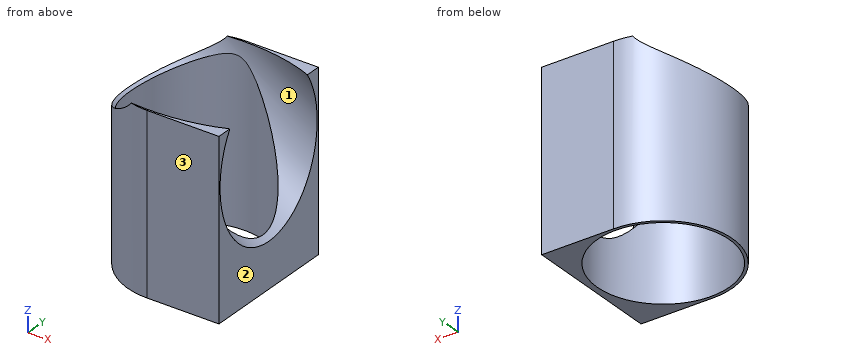
```python
from build123d import *

# Parameters (mm, degrees)
SKETCH1_R           = 23.525
SKETCH1_R_2         = 22.525
BOSS_EXTRUDE1_DEPTH = 60
BOSS_EXTRUDE2_DEPTH = 60
SKETCH2_R           = 23
CUT_EXTRUDE1_DEPTH  = 112.626209254


with BuildPart() as part:
    # Sketch1 → Boss-Extrude1 (new body)
    with BuildSketch(Plane.XY):
        with Locations((443.127496957, 0)):
            Circle(SKETCH1_R)
        with Locations((443.127496957, 0)):
            Circle(SKETCH1_R_2, mode=Mode.SUBTRACT)
    extrude(amount=-BOSS_EXTRUDE1_DEPTH)

    # Sketch3 → Boss-Extrude2 (add)
    with BuildSketch(Plane(origin=(0, 0, -60), x_dir=(-1, 0, 0), z_dir=(0, 0, -1))):
        with BuildLine():
            Line((-466.652496957, -23.525), (-443.127496957, -23.525))
            ThreePointArc((-443.127496957, -23.525), (-459.762183984, -16.634687027), (-466.652496957, 0))
            Line((-466.652496957, 0), (-466.652496957, -23.525))
        make_face()
        Polygon((-466.652496957, 23.525), (-467.652496957, 23.525), (-467.652496957, -23.525), (-466.652496957, -23.525), (-466.652496957, 0), align=None)
        with BuildLine():
            Line((-466.652496957, 23.525), (-466.652496957, 0))
            ThreePointArc((-466.652496957, 0), (-459.762183984, 16.634687027), (-443.127496957, 23.525))
            Line((-443.127496957, 23.525), (-466.652496957, 23.525))
        make_face()
    extrude(amount=-BOSS_EXTRUDE2_DEPTH)

    # Sketch2 → Cut-Extrude1 (cut, through all)
    with BuildSketch(Plane(origin=(254.325020267, 0, -174.059113982), x_dir=(0.564788358, 0, 0.825235791), z_dir=(-0.825235791, 0, 0.564788358))):
        with Locations((250.273251396, 0)):
            Circle(SKETCH2_R)
    extrude(amount=-CUT_EXTRUDE1_DEPTH, mode=Mode.SUBTRACT)


solid = part.part
```
Input: part model. Units: mm. Frame: model coordinates. Face numbers are marked on the shaded views. Coordinates: 2 decimals unless noted, no trailing zeros. Write each loop counter-clockwise with the first axis right and the second up, starting at its lowest first coordinate (ties: lowest second). Pieces come first, ordered by that corner, then holes. Notation, with made-up numbers: (0, 58.5) -> (34, 58.5) arc R20 cw to (34, 82.5) -> close; hole circle Ø3 at (82, 36.25). An arc over 180 degrees is marked (long way). Write each question's results on one line, items separated by ' | '.
Item 1: Section query C-C on y = -12. Return loops of the section in (x, z), plus the area to 3 significant figures.
Conclusion:
outline: (422.89, -60) -> (424.07, -60) -> (424.07, -10.73) -> (422.89, -9.93) -> close; (462.19, -60) -> (467.65, -60) -> (467.65, -40.56) -> (462.19, -36.82) -> close | area: 175 mm^2
Item 2: Section query A-A on y = 2. Return loops of the section in (x, z), plus the area to 3 significant figures.
Conclusion:
outline: (419.69, -60) -> (420.69, -60) -> (420.69, -12.41) -> (419.69, -11.72) -> close; (465.56, -60) -> (467.65, -60) -> (467.65, -44.55) -> (465.56, -43.12) -> close | area: 81.9 mm^2
Item 3: Mould query, pull axis Y, two halves, no side actions, for the marked faces 1, 2 and 3. Classes: +Y half, -Y half, draft (parallel to the pull), parting line (faces both ways), or undercut.
Conclusion:
face 1: undercut | face 2: draft | face 3: -Y half
Item 4: Pin query (flat end, axial travel): pin 1 Ø12 at (y, z) = (-14, -16) entering from +X; pin 2 Ø12 at (y, z) = (-11, -31.5) entering from +X; pin 3 Ø3 at (y, z) = (15, -26.5) entering from +X. Return the tip coordinate at first contact, or that it passes through.
Conclusion:
pin 1: stops at x = 432.77 | pin 2: stops at x = 464.87 | pin 3: stops at x = 427.79
Item 5: Material intervals for probe 1 along X at (y, z) = (0, -46); probe 2 along Y at (x, z) = (460, -12) (3 decimals); probe 3 along X at (y, z) = (0, -31), sorted ascending.
Conclusion:
probe 1: x = 419.6 to 420.6, 465.65 to 467.65 | probe 2: y = -23.525 to -22.997, 22.997 to 23.525 | probe 3: x = 419.6 to 420.6
